Print and shaded views of the part. All mm, measured from the part's lowest x, y and z. Round coordinates to 2 decimals unless told otherwise and drop trailing zeros. Loops run counter-clockwise (first coordinate to the right, second up) from the corner with the lowest first, then second, coordinate; pieces in that order, holes last. Notation, with made-up numbers: (19.25, 64.5) - (32.25, 64.5) arc R26 cw to (32.25, 82.5) - close; hole circle Ø9 at (74, 85). An arc over 180 degrees is marked (long way). Put each result on its own line as item: value. Start each with the question number.
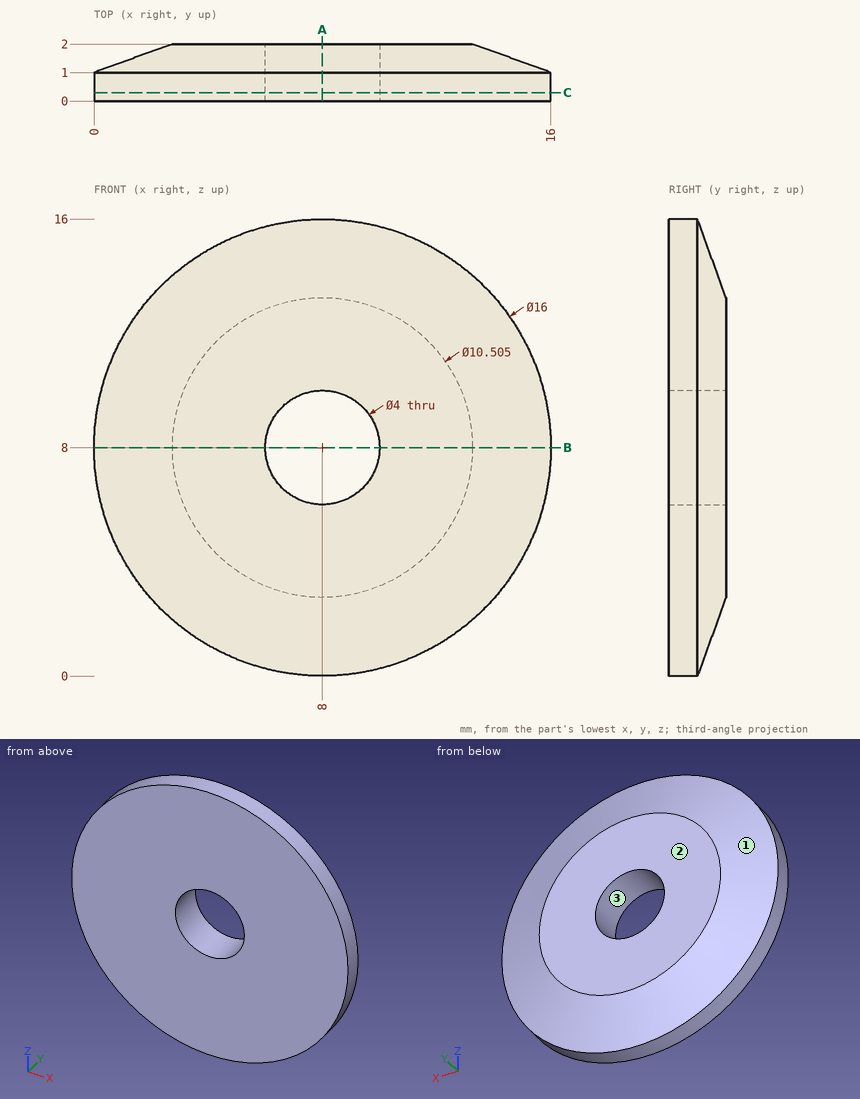
Item 1: Drill centre lines: probe 1 along Z at (x, y) = (8, 0.5); probe 2 along X at (y, z) = (0.4, 9.75). Where is each one in solid material? Low to high. Write a range as [from, to].
Item 2: Slice it at B-B (z = 8). Give the cut face in (x, y).
Item 3: Slice it at C-C (y = 0.3). Give the cut face in (x, z).
Item 4: Two-plate mould, pull along X, no slides. Class the marked faces 1, 2 and 3: pulls with the +X half, pulls with the -X half, needs draft (parallel to the pull), parting line crosses it, or undercut.
Item 5: Drop a flat-ended pin along its axis: pin 1 Ø1 at (y, z) = (1, 2) entering from +X. Give the stop position or say it passes through.
Item 6: Slice it at A-A (x = 8). Give the cut face in (y, z).
Computed values:
1. probe 1: z = [0, 6], [10, 16]
1. probe 2: x = [0.19, 7.03], [8.97, 15.81]
2. outline: (0, 0) - (6, 0) - (6, 2) - (2.75, 2) - (0, 1) - close; (10, 0) - (16, 0) - (16, 1) - (13.25, 2) - (10, 2) - close
3. outline: circle Ø16 at (8, 8); hole circle Ø4 at (8, 8)
4. face 1: parting line crosses it
4. face 2: needs draft
4. face 3: undercut
5. pin 1: stops at x = 13.81
6. outline: (0, 0) - (1, 0) - (2, 2.75) - (2, 6) - (0, 6) - close; (0, 10) - (2, 10) - (2, 13.25) - (1, 16) - (0, 16) - close
